from build123d import *

# Parameters (mm, degrees)
F2_R    = 5
F3_SIZE = 1


with BuildPart() as f1:
    # F0 (on Right) → F1 (revolve)
    with BuildSketch(Plane.YZ):
        with BuildLine():
            Line((0, 12.5), (0, 0))
            Line((0, 0), (185, 0))
            Line((185, 0), (185, 39))
            Line((185, 39), (1365, 39))
            Line((1365, 39), (1365, 0))
            Line((1365, 0), (1550, 0))
            Line((1550, 0), (1550, 12.5))
            Line((1550, 12.5), (1450, 12.5))
            Line((1450, 12.5), (1450, 45))
            Line((1450, 45), (1385, 45))
            Line((1385, 45), (1385, 38.434669))
            ThreePointArc((1385, 38.434669), (1384.786788, 38.025093), (1384.32899, 37.964823))
            Line((1384.32899, 37.964823), (1366.656932, 44.396926))
            ThreePointArc((1366.656932, 44.396926), (1364.973212, 44.848078), (1363.23673, 45))
            Line((1363.23673, 45), (187.644905, 45))
            ThreePointArc((187.644905, 45), (185.040182, 44.772116), (182.514603, 44.095389))
            Line((182.514603, 44.095389), (165.67101, 37.964823))
            ThreePointArc((165.67101, 37.964823), (165.213212, 38.025093), (165, 38.434669))
            Line((165, 38.434669), (165, 45))
            Line((165, 45), (100, 45))
            Line((100, 45), (100, 12.5))
            Line((100, 12.5), (0, 12.5))
        make_face()
    revolve(axis=Axis((0, 1457.5, 0), (0, -1, 0)))

    # F2
    f2_edges = [f1.edges().sort_by_distance(p)[0] for p in [
        (0, 1450, -12.5),
        (0, 100, -12.5),
    ]]
    fillet(f2_edges, radius=F2_R)

    # F3
    f3_edges = [f1.edges().sort_by_distance(p)[0] for p in [
        (0, 1450, -45),
        (0, 1550, -12.5),
        (0, 0, -12.5),
        (0, 100, -45),
    ]]
    chamfer(f3_edges, length=F3_SIZE)


solid = f1.part
Verification items for the finished model (mm, model axes). A direction names the side the tool comes from. Give positions to 0.01 mm unless a question says otherwise; leave off trailing zeros. Loops run counter-clockwise (first coordinate to the right, second up) from the corner with the lowest first, then second, coordinate; pieces in that order, holes last.
1) Set-up check for faces 4 (the flat face through (-20, 1385, 33)), 5 (the flat face through (19, 1450, 1)), 6 (the cylindrical face through (-3.755, 47.342, 11.923)), 7 (the cylindrical face through (39.923, 132.552, 20.765)): record each of +Z, -Z, +X, -X, +Y, -Y from which the full face is reachable in a straight line by a thin tool's end or side.
2) Depth check by flat-ended pin: pin 1 Ø1 at (y, z) = (186.5, 2.5) entering from -X; pin 2 Ø3 at (y, z) = (357, -22) entering from +X; pin 3 Ø8 at (y, z) = (978, 28) entering from +X. Enter the tip coordinate at first touch or a pass-through.
3) Thickness scan on line 1 along Z through (x, y) = (0, 691.5); line 2 along Y through (x, z) = (-36.5, -4). Record the ranges inside material, lowest first.
4) Sectioned sample at A-A, the plane y = 294. Enter the section's corners in (x, z), then the cut area to 3 significant figures.
5) Draft check along Z on faces 1 (the flat face through (-20, 165, -33)), 2 (the flat face through (-1, 1365, -1)), 3 (the cylindrical face through (-3.755, 1501.342, 11.923)). Enter one of: pulls with the +Z half, pulls with the -Z half, needs draft (parallel to the pull), parting line crosses it, or undercut.
Answers:
1. face 4: none
1. face 5: +Y
1. face 6: -Y
1. face 7: +Y, -Y
2. pin 1: stops at x = -44.93
2. pin 2: stops at x = 40.06
2. pin 3: stops at x = 38.07
3. line 1: z = -45 to -39, 39 to 45
3. line 2: y = 100 to 185, 1365 to 1450
4. outline: circle Ø90 at (0, 0); hole circle Ø78 at (0, 0)
4. area: 1,580 mm2
5. face 1: needs draft
5. face 2: undercut
5. face 3: parting line crosses it
